Verification items for the finished model (mm, model axes). A direction names the side the tool comes from. Give positions to 0.01 mm unless a question says otherwise; leave off trailing zeros. Loops run counter-clockwise (first coordinate to the right, second up) from the corner with the lowest first, then second, coordinate; pieces in that order, holes last. Notation, with made-up numbers: (-18, 10.25) -> (40, 10.25) arc R24 cw to (40, 23.25) -> close; hole circle Ø5 at (13.5, 24). An arc over 180 degrees is marked (long way). Answer in a Markdown table with one row per item. Add a question column.
Q1. Material ranges on probe 1 along Y at (x, z) = (0, 6.5); probe 2 along Z at (x, y) = (15.5, -3.5); probe 3 along Y at (x, z) = (-7, 8), recorded low to high.
Q2. Set-up check for faces 1 (the face through (-12, -11, 10)), 2 (the face through (0, -5, 2)), 3 (the face through (1.5, 12, 1)): record each of +Z, -Z, +X, -X, +Y, -Y from which the full face is reachable in a straight line by a thin tool's end or side.
Q3. Section check D-D on x = -12. Enter the section's corners in (y, z).
Q4. Release check for a two-part mould opening along Y. For faces 4 (the face through (-2.343, 17.847, 4.93)), 5 (the face through (4, -4, 0)), 6 (the face through (-6.46, -6.35, 0.99)) record: pulls with the +Y half, pulls with the -Y half, needs draft (parallel to the pull), parting line crosses it, or undercut.
Q5. Gauge pin test, flat ends, axial feed: P1, Ø0.6, axis at y = -12, z = 0.5, coming from the +X side; P2, Ø5, axis at x = 3, z = 2, coming from the +Y side; P3, Ø0.6, axis at x = 12, z = 0.5, coming from the -Y side; P4, Ø2, axis at x = 9, y = -12.5, coming from the -Z side. Record the tip position at first contact, or that the pin passes through.
Q6. Section check C-C on y = -8.5. Enter the section's corners in (x, z), and give its area (3 significant figures).
Q7. Section check A-A on y = 0. Enter the section's corners in (x, z).
```python
from build123d import *

# Parameters (mm, degrees)
ESBO_O1_R                = 16
ESBO_O1_R_2              = 4.15
RESSALTO_EXTRUS_O1_DEPTH = 2
ESBO_O2_R                = 18
ESBO_O2_R_2              = 16
RESSALTO_EXTRUS_O2_DEPTH = 10
CORTE_EXTRUS_O1_DEPTH    = 10


with BuildPart() as part:
    # Esboço1 → Ressalto-extrusão1 (new body)
    with BuildSketch(Plane.XY):
        Circle(ESBO_O1_R)
        Circle(ESBO_O1_R_2, mode=Mode.SUBTRACT)
    extrude(amount=RESSALTO_EXTRUS_O1_DEPTH)

    # Esboço2 → Ressalto-extrusão2 (add)
    with BuildSketch(Plane.XY):
        Circle(ESBO_O2_R)
        Circle(ESBO_O2_R_2, mode=Mode.SUBTRACT)
    extrude(amount=RESSALTO_EXTRUS_O2_DEPTH)

    # Esboço3 → Corte-extrusão1 (cut)
    with BuildSketch(Plane(origin=(0, 0, 0), x_dir=(-1, 0, 0), z_dir=(0, 0, -1))):
        with BuildLine():
            ThreePointArc((-1.5, -8.932222345), (-6.404474843, -6.404474843), (-8.932222345, -1.5))
            Line((-8.932222345, -1.5), (-15.344338178, -1.5))
            ThreePointArc((-15.344338178, -1.5), (-10.90180522, -10.90180522), (-1.5, -15.344338178))
            Line((-1.5, -15.344338178), (-1.5, -8.932222345))
        make_face()
        with BuildLine():
            ThreePointArc((8.932222345, -1.5), (6.404474843, -6.404474843), (1.5, -8.932222345))
            Line((1.5, -8.932222345), (1.5, -15.344338178))
            ThreePointArc((1.5, -15.344338178), (10.90180522, -10.90180522), (15.344338178, -1.5))
            Line((15.344338178, -1.5), (8.932222345, -1.5))
        make_face()
        with BuildLine():
            ThreePointArc((1.5, 8.932222345), (6.404474843, 6.404474843), (8.932222345, 1.5))
            Line((8.932222345, 1.5), (15.344338178, 1.5))
            ThreePointArc((15.344338178, 1.5), (10.90180522, 10.90180522), (1.5, 15.344338178))
            Line((1.5, 15.344338178), (1.5, 8.932222345))
        make_face()
        with BuildLine():
            ThreePointArc((-8.932222345, 1.5), (-6.404474843, 6.404474843), (-1.5, 8.932222345))
            Line((-1.5, 8.932222345), (-1.5, 15.344338178))
            ThreePointArc((-1.5, 15.344338178), (-10.90180522, 10.90180522), (-15.344338178, 1.5))
            Line((-15.344338178, 1.5), (-8.932222345, 1.5))
        make_face()
    extrude(amount=-CORTE_EXTRUS_O1_DEPTH, mode=Mode.SUBTRACT)


solid = part.part
```
Taken from the geometry:
| question | item | result |
|---|---|---|
| 1 | probe 1 | y = -18 to -16, 16 to 18 |
| 1 | probe 2 | z = 0 to 2 |
| 1 | probe 3 | y = -16.58 to -14.39, 14.39 to 16.58 |
| 2 | face 1 | +Z, +X, -X, +Y, -Y |
| 2 | face 2 | +Z |
| 2 | face 3 | +Z, -Z |
| 3 | outline | (-13.42, 0) -> (-9.68, 0) -> (-9.68, 2) -> (-10.58, 2) -> (-10.58, 10) -> (-13.42, 10) -> close; (-1.5, 0) -> (1.5, 0) -> (1.5, 2) -> (-1.5, 2) -> close; (9.68, 0) -> (13.42, 0) -> (13.42, 10) -> (10.58, 10) -> (10.58, 2) -> (9.68, 2) -> close |
| 4 | face 4 | parting line crosses it |
| 4 | face 5 | needs draft |
| 4 | face 6 | undercut |
| 5 | P1 | stops at x = 13.68 |
| 5 | P2 | stops at y = 17.99 |
| 5 | P3 | stops at y = -13.68 |
| 5 | P4 | stops at z = 0 |
| 6 | outline | (-15.87, 0) -> (-12.86, 0) -> (-12.86, 2) -> (-13.56, 2) -> (-13.56, 10) -> (-15.87, 10) -> close; (-3.13, 0) -> (3.13, 0) -> (3.13, 2) -> (-3.13, 2) -> close; (12.86, 0) -> (15.87, 0) -> (15.87, 10) -> (13.56, 10) -> (13.56, 2) -> (12.86, 2) -> close |
| 6 | area | 61.5 mm² |
| 7 | outline | (-18, 0) -> (-4.15, 0) -> (-4.15, 2) -> (-16, 2) -> (-16, 10) -> (-18, 10) -> close; (4.15, 0) -> (18, 0) -> (18, 10) -> (16, 10) -> (16, 2) -> (4.15, 2) -> close |
